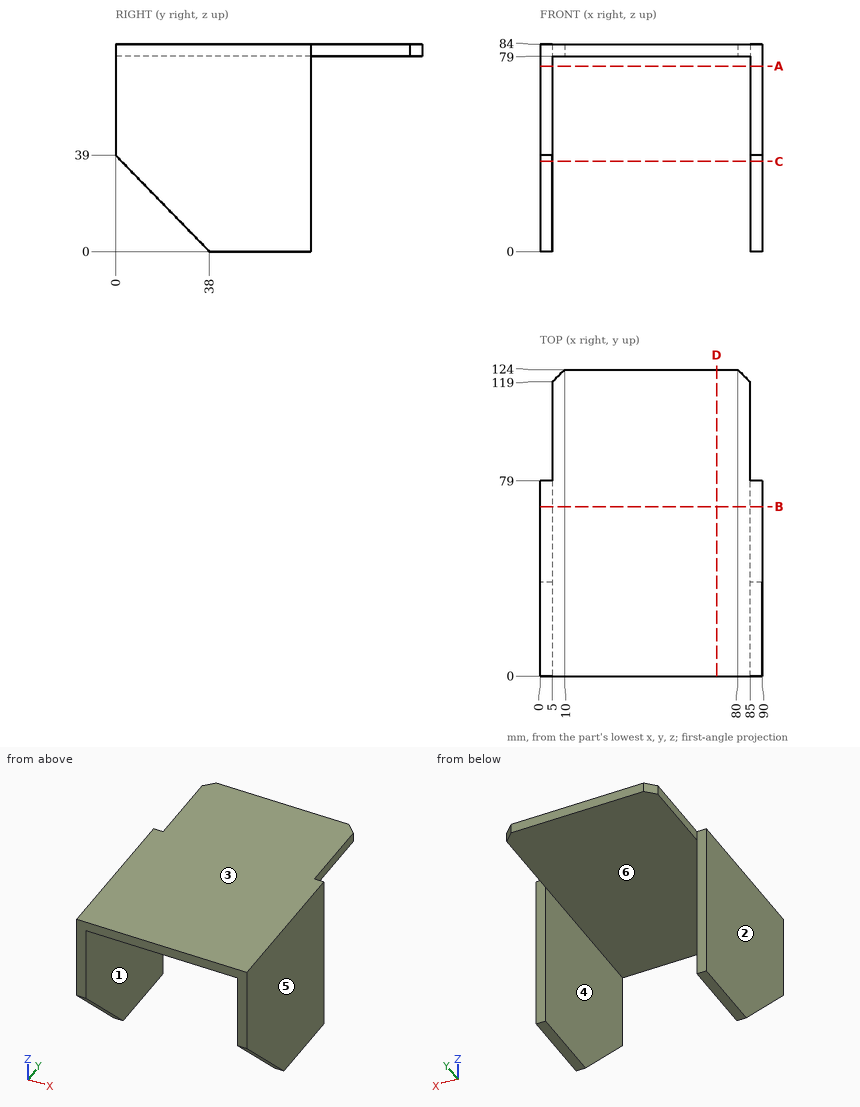
Design review of the part shown in the three views and the two pictorial views. Dimensions are in mm from the part's minimum x, y and z. A direction names the side the tool comes from. Give positions to 0.01 mm unless a question says otherwise; leave off trailing zeros. Loops run counter-clockwise (first coordinate to the right, second up) from the corner with the lowest first, then second, coordinate; pieces in that order, holes last. Notation, with made-up numbers: (60, -31) -> (90, -31) arc R11 cw to (90, -10) -> close; hole circle Ø9 at (34.5, 59.25). An arc over 180 degrees is marked (long way). Put each result on its own line as item: value. Start each with the question number.
1. We need section C-C on z = 36.5. State the section outline as (x, y) points, then the cut area to 3 significant figures.
2. Wall thickness on probe 1 along X at (y, z) = (44.5, 8.5); probe 2 along Z at (x, y) = (36, 84.5): over which ranges is each line inside the solid? List them lowest first.
3. Mouldability with a two-part tool opening along X and no side actions: class the marked faces 3, 4, 5 and 6 as released by +X, released by -X, zero draft, split by the parting line, or undercut.
4. We need section A-A on z = 75. State the section outline as (x, y) points, then the cut area to 3 significant figures.
5. We need section D-D on x = 71.5. State the section outline as (y, z) points, then the cut area to 3 significant figures.
6. For the marked faces 1 and 2, list the 3-axis set-ups (+Z, -Z, +X, -X, +Y, -Y) from which the entire face can be reached by the end or side of a thin tool; tool diameter is ignored.
7. We need section B-B on y = 68.5. State the section outline as (x, z) points.
8. Clearance check with flat-ended pins moving along their axes: P1, Ø4, axis at y = 91.5, z = 80.5, coming from the -X side; P2, Ø23.5, axis at y = 25, z = 57, coming from the -X side; P3, Ø4, axis at x = 2, z = 46.5, coming from the +Y side; P4, Ø8, axis at x = 72.5, z = 73, coming from the +Y side. State where each tip first meets the part, or that it passes through.
Determined:
1. outline: (0, 2.44) -> (5, 2.44) -> (5, 79) -> (0, 79) -> close; (85, 2.44) -> (90, 2.44) -> (90, 79) -> (85, 79) -> close
1. area: 766 mm^2
2. probe 1: 0 to 5, 85 to 90
2. probe 2: 79 to 84
3. face 3: zero draft
3. face 4: undercut
3. face 5: released by +X
3. face 6: undercut
4. outline: (0, 0) -> (5, 0) -> (5, 79) -> (0, 79) -> close; (85, 0) -> (90, 0) -> (90, 79) -> (85, 79) -> close
4. area: 790 mm^2
5. outline: (0, 79) -> (124, 79) -> (124, 84) -> (0, 84) -> close
5. area: 620 mm^2
6. face 1: -Z, +Y, -Y
6. face 2: +Z, -Z, -X, +Y, -Y
7. outline: (0, 0) -> (5, 0) -> (5, 79) -> (85, 79) -> (85, 0) -> (90, 0) -> (90, 84) -> (0, 84) -> close
8. P1: x = 5
8. P2: x = 0
8. P3: y = 79
8. P4: through
